from build123d import *

# Parameters (mm, degrees)
SKETCH1_R                         = 30.48
MAIN_BODY_EXTRUDE_DEPTH           = 15.24
THROUGH_HOLE_FOR_BLOOD_DEPTH      = 46.72
THROUGH_HOLE_FOR_BLOOD_DEPTH_BACK = 46.72
SKETCH2_R                         = 10.16
M5_CLEARANCE_HOLE_D               = 5.5
SCREW_HOLE_PATTERN_COUNT          = 4
CUT_EXTRUDE2_DEPTH                = 46.72
SKETCH18_7_R                      = 2.5908
FLAT_SIDE_DOWEL_HOLE_DEPTH        = 3.81
SKETCH27_4_R                      = 2.54
FLAT_SIDE_DOWEL_DEPTH             = 3.81
CIRPATTERN1_COUNT                 = 2
CIRPATTERN2_COUNT                 = 2
SKETCH52_R                        = 12.7
SKETCH52_R_2                      = 10.16
REVOLVE2_ANGLE                    = 8
F_1_4_28_TAPPED_HOLE1_REACH       = 77.996
F_1_4_28_TAPPED_HOLE1_BORE_R      = 2.7051


with BuildPart() as part:
    # Sketch1 → Main Body Extrude (new body)
    with BuildSketch(Plane(origin=(0, 0, 0), x_dir=(1, 0, 0), z_dir=(0, 1, 0))):
        with Locations(Location((0, 0, 0), (0, 0, 90))):
            Circle(SKETCH1_R)
    extrude(amount=MAIN_BODY_EXTRUDE_DEPTH)

    # Sketch2 → Through Hole For Blood (cut, two sides: drawn at the far end of the back side and taken through both)
    with BuildSketch(Plane(origin=(0, 15.24, 0), x_dir=(1, 0, 0), z_dir=(0, 1, 0)).offset(-THROUGH_HOLE_FOR_BLOOD_DEPTH_BACK)):
        with Locations(Location((0, 0, 0), (0, 0, 270))):
            Circle(SKETCH2_R)
    extrude(amount=THROUGH_HOLE_FOR_BLOOD_DEPTH + THROUGH_HOLE_FOR_BLOOD_DEPTH_BACK, mode=Mode.SUBTRACT)

    # M5 Clearance Hole (through all)
    with Locations(Plane(origin=(0, 0, 0), x_dir=(-1, 0, 0), z_dir=(0, -1, 0))):
        with Locations((17.06248663, -17.06248663)):
            m5_clearance_hole = Hole(M5_CLEARANCE_HOLE_D / 2)

    # Screw Hole Pattern: M5 Clearance Hole ×4 about axis
    screw_hole_pattern_axis = Axis((0, 0, 0), (0, 1, 0))
    for i in range(1, SCREW_HOLE_PATTERN_COUNT):
        add(m5_clearance_hole.rotate(screw_hole_pattern_axis, i * 360 / SCREW_HOLE_PATTERN_COUNT), mode=Mode.SUBTRACT)

    # Sketch42 → Cut-Extrude2 (cut, through all)
    with BuildSketch(Plane.XZ):
        with BuildLine():
            Line((27.708128771, 12.7), (27.708128771, -12.7))
            ThreePointArc((27.708128771, -12.7), (30.48, 0), (27.708128771, 12.7))
        make_face()
    extrude(amount=-CUT_EXTRUDE2_DEPTH, mode=Mode.SUBTRACT)

    # Sketch18<7> → Flat Side Dowel Hole (cut)
    with BuildSketch(Plane(origin=(0, 0, 0), x_dir=(-1, 0, 0), z_dir=(0, -1, 0))):
        with Locations(Location((-21.741151963, 7.064128491, 0), (0, 0, 90))):
            Circle(SKETCH18_7_R)
    flat_side_dowel_hole = extrude(amount=-FLAT_SIDE_DOWEL_HOLE_DEPTH, mode=Mode.SUBTRACT)

    # Sketch27<4> → Flat Side Dowel (add)
    with BuildSketch(Plane.XZ):
        with Locations(Location((0, 22.86, 0), (0, 0, 90))):
            Circle(SKETCH27_4_R)
    flat_side_dowel = extrude(amount=FLAT_SIDE_DOWEL_DEPTH)

    # CirPattern1: Flat Side Dowel Hole ×2 about axis
    cirpattern1_axis = Axis((0, 0, 0), (0, 1, 0))
    for i in range(1, CIRPATTERN1_COUNT):
        add(flat_side_dowel_hole.rotate(cirpattern1_axis, i * 360 / CIRPATTERN1_COUNT), mode=Mode.SUBTRACT)

    # CirPattern2: Flat Side Dowel ×2 about axis
    cirpattern2_axis = Axis((0, 0, 0), (0, 1, 0))
    for i in range(1, CIRPATTERN2_COUNT):
        add(flat_side_dowel.rotate(cirpattern2_axis, i * 360 / CIRPATTERN2_COUNT))

    # Sketch52 → Revolve2 (revolve)
    with BuildSketch(Plane(origin=(0, 15.24, 0), x_dir=(1, 0, 0), z_dir=(0, 1, 0))):
        Circle(SKETCH52_R)
        with Locations(Location((0, 0, 0), (0, 0, 270))):
            Circle(SKETCH52_R_2, mode=Mode.SUBTRACT)
    revolve(axis=Axis((0, 15.24, 152.4), (1, 0, 0)), revolution_arc=REVOLVE2_ANGLE)

    # 1/4-28 Tapped Hole1 bore → 1/4-28 Tapped Hole1 (cut, up to next)
    with BuildSketch(Plane(origin=(27.708128771, 0, 0), x_dir=(0, 0, -1), z_dir=(1, 0, 0)), mode=Mode.PRIVATE) as f_1_4_28_tapped_hole1_sk1:
        with Locations((0, 7.62)):
            Circle(F_1_4_28_TAPPED_HOLE1_BORE_R)
    f_1_4_28_tapped_hole1_tool1 = extrude(f_1_4_28_tapped_hole1_sk1.sketch, amount=-F_1_4_28_TAPPED_HOLE1_REACH, mode=Mode.PRIVATE) & part.part
    add(f_1_4_28_tapped_hole1_tool1.solids().sort_by_distance((27.708129, 7.62, 0))[0], mode=Mode.SUBTRACT)


solid = part.part
Work out the finished part from the listing and answer in its coordinate system (mm). A direction names the side the tool comes from. Round coordinates to 2 decimals unless told otherwise and drop trailing zeros. Write each loop counter-clockwise with the first axis right and the second up, starting at its lowest first coordinate (ties: lowest second). Pieces come first, ordered by that corner, then holes. Notation, with made-up numbers: M -39,4 L -23,4 A25 ccw -23,22 Z; hole C 33.25,87.25 d1. An arc over 180 degrees is marked long. Use a Markdown table: item, result.
1) The part is cut by section D-D on y = 7.62. Give the vertices of the cut face in (x, z).
Taken from the geometry:
| item | result |
|---|---|
| outline | M 9.79,-2.71 A10.16 cw long 9.79,2.71 L 27.71,2.71 L 27.71,12.7 A30.48 ccw long 27.71,-12.7 L 27.71,-2.71 Z; hole C -17.06,-17.06 d5.5; hole C -17.06,17.06 d5.5; hole C 17.06,-17.06 d5.5; hole C 17.06,17.06 d5.5 |
2) Flat-ended cylindrical pins translate along their axes: pin 1 (4 mm diameter, centred on x = -14.5, y = 0.5, fed in from -Z); pin 2 (17.5 mm diameter, centred on x = 5.5, z = -1, fed in from -Y); pin 3 (4 mm diameter, centred on x = -21.74, z = 7.06, fed in from -Y); pin 4 (5 mm diameter, centred on x = 17.06, z = 17.06, fed in from -Y). Find the tip coordinate at first contact, or state that the pin passes through.
Taken from the geometry:
| item | result |
|---|---|
| pin 1 | stops at z = -27.8 |
| pin 2 | stops at y = 0 |
| pin 3 | stops at y = 3.81 |
| pin 4 | passes through |
3) The part is cut by section C-C on z = -18. Give the vertices of the cut face in (x, y).
Taken from the geometry:
| item | result |
|---|---|
| outline | M -24.6,0 L -19.65,0 L -19.65,15.24 L -24.6,15.24 Z; M -14.48,0 L 14.48,0 L 14.48,15.24 L -14.48,15.24 Z; M 19.65,0 L 24.6,0 L 24.6,15.24 L 19.65,15.24 Z |
4) Determine the mould class of faces 1 (the face through (-14.522, 7.727, 18.116)), 2 (the face through (-30.458, 7.513, -1.157)), 3 (the face through (0, -3.81, 23)) for opening direction X: pulls with the +X half, pulls with the -X half, needs draft (parallel to the pull), parting line crosses it, or undercut.
Taken from the geometry:
| item | result |
|---|---|
| face 1 | undercut |
| face 2 | parting line crosses it |
| face 3 | needs draft |
5) The part is cut by section B-B on y = 1. Give the vertices of the cut face in (x, z).
Taken from the geometry:
| item | result |
|---|---|
| outline | M 27.71,-12.7 L 27.71,12.7 A30.48 ccw long Z; hole C -21.74,7.06 d5.18; hole C -17.06,-17.06 d5.5; hole C -17.06,17.06 d5.5; hole C 0,0 d20.32; hole C 17.06,-17.06 d5.5; hole C 17.06,17.06 d5.5; hole C 21.74,-7.06 d5.18 |
6) Which of the six approach directions +Z, -Z, +X, -X, +Y, -Y give full straight-line access (tool end or side, diameter ignored) to faces 4 (the face through (-0.112, -1.878, 20.322)), 5 (the face through (14.522, 7.727, -18.116)), 6 (the face through (18.876, 9.901, -1.454))?
Taken from the geometry:
| item | result |
|---|---|
| face 4 | -Y |
| face 5 | +Y, -Y |
| face 6 | +X |
7) The part is cut by section A-A on x = 0. Give the vertices of the cut face in (y, z).
Taken from the geometry:
| item | result |
|---|---|
| outline | M -3.81,-25.4 L 0,-25.4 L 0,-30.48 L 15.24,-30.48 L 15.24,-12.7 A165.1 ccw 38.22,-11.09 L 37.86,-8.58 A162.56 cw 15.24,-10.16 L 0,-10.16 L 0,-20.32 L -3.81,-20.32 Z; M -3.81,20.32 L 0,20.32 L 0,10.16 L 15.24,10.16 A142.24 ccw 35.04,11.54 L 34.68,14.06 A139.7 cw 15.24,12.7 L 15.24,30.48 L 0,30.48 L 0,25.4 L -3.81,25.4 Z |
8) Consider line 1 (Z direction, x = 0, y = 5.75); line 2 (Z direction, x = -18.5, y = 5); line 3 (X direction, y = 9.75, z = 0). Determine where each line is inside the solid, lowest interval first. Write a range as [from, to].
Taken from the geometry:
| item | result |
|---|---|
| line 1 | z = [-30.48, -10.16], [10.16, 30.48] |
| line 2 | z = [-24.22, -19.41], [-14.72, 14.72], [19.41, 24.22] |
| line 3 | x = [-30.48, -10.16] |
